from build123d import *
from build123d.topology import SkipClean

# Parameters (mm, degrees)
SKETCH4_W                = 28
SKETCH4_H                = 28
CUT_EXTRUDE1_DEPTH       = 9.05
SKETCH5_W                = 2.5
SKETCH5_H                = 6
REVOLVE3_ANGLE           = 12.5
REVOLVE3_OTHER_WAY_ANGLE = 12.5
SKETCH6_W                = 2.5
SKETCH6_H                = 6
REVOLVE4_ANGLE           = 12.5
REVOLVE4_OTHER_WAY_ANGLE = 12.5
SKETCH7_R                = 1.5875
CUT_EXTRUDE2_DEPTH       = 38.666032443


with BuildPart() as part:
    # Sketch1 → Revolve1 (revolve)
    with BuildSketch(Plane.XY, mode=Mode.PRIVATE) as revolve1_sk:
        Polygon((0, 0), (-7, 0), (-7.7, 0.7), (-7.7, 8.325), (-6.975, 9.05), (-6.25, 9.05), (-5.625, 10.136), (-5.625, 10.436), (-6.25, 10.936), (-6.25, 11.66), (-5.75, 12.16), (-4.375, 12.16), (-4.375, 17.16), (-5.75, 17.16), (-6.25, 17.66), (-6.25, 28.642), (-5.625, 28.942), (-5.625, 29.242), (-5, 29.242), (-5, 29.442), (-5.625, 29.442), (-5.625, 29.877538462), (-5, 30.166), (-3.6, 30.166), (-3.6, 30.89), (-6.25, 30.89), (-6.25, 32.7), (0, 32.7), align=None)
    revolve(revolve1_sk.sketch.rotate(Axis((0, 32.7, 0), (0, -1, 0)), 90), axis=Axis((0, 32.7, 0), (0, -1, 0)))

    # Sketch2 → Revolve2 (revolve)
    with BuildSketch(Plane.XY, mode=Mode.PRIVATE) as revolve2_sk:
        Polygon((0, -3.5), (-2.0095, -3.5), (-2.5, -3.0095), (-2.5, -0.5), (-4.2, -0.5), (-4.2, 0), (0, 0), align=None)
    revolve(revolve2_sk.sketch.rotate(Axis((0, 0, 0), (0, -1, 0)), 90), axis=Axis((0, 0, 0), (0, -1, 0)))

    # Sketch3 → Cut-Revolve1 (revolve, cut)
    with BuildSketch(Plane.XY, mode=Mode.PRIVATE) as cut_revolve1_sk:
        Polygon((0, -3.5), (-1.25, -3.5), (-1.25, 1), (-3, 1), (-3, 32.7), (0, 32.7), align=None)
    revolve(cut_revolve1_sk.sketch.rotate(Axis((0, 32.7, 0), (0, -1, 0)), 90), axis=Axis((0, 32.7, 0), (0, -1, 0)), mode=Mode.SUBTRACT)

    # Sketch4 → Cut-Extrude1 (cut)
    with BuildSketch(Plane(origin=(0, 0, 0), x_dir=(-1, 0, 0), z_dir=(0, 1, 0))):
        Rectangle(SKETCH4_W, SKETCH4_H)
        Polygon((8.082903769, 0), (4.041451884, 7), (-4.041451884, 7), (-8.082903769, 0), (-4.041451884, -7), (4.041451884, -7), align=None, mode=Mode.SUBTRACT)
    extrude(amount=CUT_EXTRUDE1_DEPTH, mode=Mode.SUBTRACT)

    # Sketch5 → Revolve3 (revolve)
    with BuildSketch(Plane(origin=(0, 0, 0), x_dir=(0, 0, -1), z_dir=(1, 0, 0))):
        with Locations((5, 14.66)):
            Rectangle(SKETCH5_W, SKETCH5_H)
    revolve(axis=Axis((0, 11.66, 0), (0, 1, 0)), revolution_arc=REVOLVE3_ANGLE)

    # Sketch5 → Revolve3 other way (revolve)
    with BuildSketch(Plane(origin=(0, 0, 0), x_dir=(0, 0, -1), z_dir=(1, 0, 0))):
        with Locations((5, 14.66)):
            Rectangle(SKETCH5_W, SKETCH5_H)
    revolve(axis=Axis((0, 11.66, 0), (0, -1, 0)), revolution_arc=REVOLVE3_OTHER_WAY_ANGLE)

    # Sketch6 → Revolve4 (revolve)
    with SkipClean():  # the faces are left unmerged after this step: merging them gives an invalid solid
        with BuildSketch(Plane(origin=(0, 0, 0), x_dir=(0, 0, -1), z_dir=(1, 0, 0))):
            with Locations((-5, 14.66)):
                Rectangle(SKETCH6_W, SKETCH6_H)
        revolve(axis=Axis((0, 17.66, 0), (0, -1, 0)), revolution_arc=REVOLVE4_ANGLE)

    # Sketch6 → Revolve4 other way (revolve)
    with SkipClean():  # the faces are left unmerged after this step: merging them gives an invalid solid
        with BuildSketch(Plane(origin=(0, 0, 0), x_dir=(0, 0, -1), z_dir=(1, 0, 0))):
            with Locations((-5, 14.66)):
                Rectangle(SKETCH6_W, SKETCH6_H)
        revolve(axis=Axis((0, 17.66, 0), (0, 1, 0)), revolution_arc=REVOLVE4_OTHER_WAY_ANGLE)

    # Sketch7 → Cut-Extrude2 (cut, through all)
    with SkipClean():  # the faces are left unmerged after this step: merging them gives an invalid solid
        with BuildSketch(Plane.XZ.offset(3.5)):
            with Locations(Location((0, 0, 0), (0, 0, 270))):
                Circle(SKETCH7_R)
        extrude(amount=-CUT_EXTRUDE2_DEPTH, mode=Mode.SUBTRACT)


solid = part.part
Geometry check sheet. Reference: the model listing, model coordinates, mm. A direction names the side the tool comes from. Coordinates: 2 decimals unless noted, no trailing zeros. Order: outer loops, then holes, each group sorted by start corner. A loop starts at its lowest first (then second) coordinate and runs counter-clockwise, first axis right, second up. Notation, with made-up numbers: (-29, 85) -> (-7, 85) arc R24 ccw to (-7, 95) -> close; hole circle Ø5 at (10.25, 67). An arc over 180 degrees is marked (long way). Use a Markdown table: item, result. Add a question column.
1. Cross-section at A-A (y = 21.5). Enter the section's corners in (x, z), and give its area (3 significant figures).
2. Material ranges on L1, parallel to X at y = -1.4, z = 0; L2, parallel to X at y = 21, z = 0; L3, parallel to Y at x = 4.75, z = 0.5, recorded low to high.
3. Go/stop test with flat-tipped pins: pin 1 Ø1.5 at (y, z) = (23.5, 4.5) entering from -X; pin 2 Ø2 at (x, z) = (-5.5, 5) entering from +Y; pin 3 Ø8 at (y, z) = (14.5, 2.5) entering from +X. Record where each tip stops, or that it passes through.
4. Mould release check, pull along X, two halves, no side actions. Record for faces 6 (the face through (-3.645, 0.199, -6.208)), 7 (the face through (3.645, 0.199, 6.208)), 8 (the face through (0.9, 17.07, -2.86)), 9 (the face through (1.081, 30.533, -3.434)): pulls with the +X half, pulls with the -X half, needs draft (parallel to the pull), parting line crosses it, or undercut.
5. Set-up check for faces 1 (the face through (-1.153, 14.702, 5.199)), 2 (the face through (0.1, -1.7, 2.5)), 3 (the face through (4.374, 14.695, -0.083)), 4 (the face through (-6.04, 4.45, -3.54)), 5 (the face through (-1.3, 1, 1.3)): record each of +Z, -Z, +X, -X, +Y, -Y from which the full face is reachable in a straight line by a thin tool's end or side.
6. Cross-section at B-B (y = 9.5). Enter the section's corners in (x, z), and give its area (3 significant figures).
Filled sheet:
| question | item | result |
|---|---|---|
| 1 | outline | circle Ø12.5 at (0, 0); hole circle Ø6 at (0, 0) |
| 1 | area | 94.4 mm2 |
| 2 | L1 | -2.5 to -1.59, 1.59 to 2.5 |
| 2 | L2 | -6.25 to -3, 3 to 6.25 |
| 2 | L3 | 0 to 12.16, 17.16 to 30.17, 30.89 to 32.7 |
| 3 | pin 1 | x = -5 |
| 3 | pin 2 | y = 9.05 |
| 3 | pin 3 | x = 6.25 |
| 4 | face 6 | pulls with the -X half |
| 4 | face 7 | pulls with the +X half |
| 4 | face 8 | undercut |
| 4 | face 9 | parting line crosses it |
| 5 | face 1 | -X |
| 5 | face 2 | -Y |
| 5 | face 3 | +X |
| 5 | face 4 | -Z, -X, +Y, -Y |
| 5 | face 5 | +Y |
| 6 | outline | circle Ø11.98 at (0, 0); hole circle Ø6 at (0, 0) |
| 6 | area | 84.5 mm2 |
